```python
from build123d import *

# Parameters (mm, degrees)
BOSS_EXTRUDE1_DEPTH = 6.08
BOSS_EXTRUDE2_DEPTH = 6.09
SKETCH4_W           = 70.899698082
SKETCH4_H           = 9.313865989
CUT_EXTRUDE4_DEPTH  = 13.09
SKETCH5_W           = 29.305939782
SKETCH5_H           = 12.234342693
CUT_EXTRUDE5_DEPTH  = 19.09
SKETCH6_R           = 6
CUT_EXTRUDE6_DEPTH  = 60.839839878
CUT_EXTRUDE7_DEPTH  = 11.09
SKETCH10_W          = 36.097359295
SKETCH10_H          = 22.987225517
CUT_EXTRUDE11_DEPTH = 63.929843377
SKETCH12_W          = 7.8
SKETCH12_H          = 6.08
BOSS_EXTRUDE4_DEPTH = 6
CUT_EXTRUDE12_REACH = 66.913
SKETCH13_W          = 18.746233403
SKETCH13_H          = 9.142839949


with BuildPart() as part:
    # Sketch1 → Boss-Extrude1 (new body)
    with BuildSketch(Plane(origin=(0, 0, 0), x_dir=(1, 0, 0), z_dir=(0, 1, 0))):
        Polygon((-14.914047624, 10.796093069), (-14.914047624, -10.733906931), (57.585952376, -8.821379846), (57.585952376, 8.878620154), align=None)
    extrude(amount=BOSS_EXTRUDE1_DEPTH)

    # Sketch2 → Boss-Extrude2 (add)
    with BuildSketch(Plane(origin=(0, 6.08, 0), x_dir=(1, 0, 0), z_dir=(0, 1, 0))):
        Polygon((-13.064047624, 10.74716445), (-13.064047624, -1.521917904), (57.585952376, 0.341806766), (57.585952376, 8.878620154), align=None)
    extrude(amount=BOSS_EXTRUDE2_DEPTH)

    # Sketch4 → Cut-Extrude4 (cut)
    with BuildSketch(Plane(origin=(0.078934537, 1.089467811, 2.992247256), x_dir=(0.9996522376299903, 0, -0.026370510070028146), z_dir=(0.02478017371916596, 0.34202014332566605, 0.9393658310530242))):
        with Locations((22.35021085, 9.967746424)):
            Rectangle(SKETCH4_W, SKETCH4_H)
    extrude(amount=CUT_EXTRUDE4_DEPTH, mode=Mode.SUBTRACT)

    # Sketch5 → Cut-Extrude5 (cut)
    with BuildSketch(Plane(origin=(52.803749931, 19.218993233, 0), x_dir=(0, 0, -1), z_dir=(0.9396926207859081, 0.34202014332566943, 1.2295842975475839e-15))):
        with Locations((0.411188199, -7.865053205)):
            Rectangle(SKETCH5_W, SKETCH5_H)
    extrude(amount=CUT_EXTRUDE5_DEPTH, mode=Mode.SUBTRACT)

    # Sketch6 → Cut-Extrude6 (cut, through all)
    with BuildSketch(Plane.XZ):
        with Locations((27.215952376, 13.62392238)):
            Circle(SKETCH6_R)
        with Locations((27.215952376, -13.683241685)):
            Circle(SKETCH6_R)
        Polygon((-14.914047624, 10.733906931), (-14.914047624, 8.733906931), (-12.914047624, 10.681147563), align=None)
        Polygon((-14.914047624, -10.796093069), (-12.914047624, -10.743197265), (-14.914047624, -8.796093069), align=None)
        Polygon((55.586647901, 8.874120866), (57.585952376, 8.821379846), (57.585952376, 6.821379846), align=None)
        Polygon((57.585952376, -8.878620154), (57.585952376, -6.878620154), (55.585952376, -8.931515959), align=None)
    extrude(amount=-CUT_EXTRUDE6_DEPTH, mode=Mode.SUBTRACT)

    # Sketch7 → Cut-Extrude7 (cut)
    with BuildSketch(Plane(origin=(0.305261026, 5.260141687, -11.541974951), x_dir=(-0.9997105289622884, 0.009976365195544153, -0.021893615951381312), z_dir=(0.024059473814631405, 0.4145836859950284, -0.9096930850712998))):
        Polygon((-26.921663821, 7.88786599), (-26.921663821, 3.064364781), (-63.575410801, 3.466220434), (-63.575410801, 10.38968732), (-26.921663821, 9.987831666), align=None)
    extrude(amount=CUT_EXTRUDE7_DEPTH, mode=Mode.SUBTRACT)

    # Sketch10 → Cut-Extrude11 (cut, through all)
    with BuildSketch(Plane.ZY.offset(3.214047624)):
        with Locations((0.41938451, 3.731019242)):
            Rectangle(SKETCH10_W, SKETCH10_H)
    extrude(amount=CUT_EXTRUDE11_DEPTH, mode=Mode.SUBTRACT)

    # Sketch12 → Boss-Extrude4 (add)
    with BuildSketch(Plane.ZY.offset(3.214047624)):
        with Locations((-0.030693992, 3.04)):
            Rectangle(SKETCH12_W, SKETCH12_H)
    extrude(amount=BOSS_EXTRUDE4_DEPTH)

    # Sketch13 → Cut-Extrude12 (cut, up to next)
    with BuildSketch(Plane(origin=(-5.91505424, 8.447572923, 0), x_dir=(0, 0, 1), z_dir=(-0.5735764363510444, 0.819152044288993, 0)), mode=Mode.PRIVATE) as cut_extrude12_sk1:
        with Locations((-4.290942315, 4.9788615)):
            Rectangle(SKETCH13_W, SKETCH13_H)
    cut_extrude12_tool1 = extrude(cut_extrude12_sk1.sketch, amount=CUT_EXTRUDE12_REACH, mode=Mode.PRIVATE) & part.part
    add(cut_extrude12_tool1.solids().sort_by_distance((-1.83661, 11.303331, -4.290942))[0], mode=Mode.SUBTRACT)


solid = part.part
```
Model file for the job. Use its own axes, mm. A direction names the side the tool comes from. Coordinates: 2 decimals unless noted, no trailing zeros. Loops run counter-clockwise (first coordinate to the right, second up) from the corner with the lowest first, then second, coordinate; pieces in that order, holes last. Notation, with made-up numbers: (-35.75, 40) - (1.25, 40) arc R26 ccw to (1.25, 57) - close; hole circle Ø5 at (13.25, -7.5). An arc over 180 degrees is marked (long way). Write item = value, one per line. Start each with the question number.
Item 1: Saw through at B-B, the plane y = 5. List the corners of the cut face in (x, z), then the cut area to 3 significant figures.
Item 2: Saw through at A-A, the plane z = -6.25. List the corners of the cut face in (x, y), then the cut area to 3 significant figures.
Item 3: Wall check: probe 1 along Y at (x, z) = (1, 7); probe 2 along X at (y, z) = (3.25, 8.5); probe 3 along Z at (x, y) = (47.5, 3.75). Give the ranges that are in metal, low to high. Write a range as [from, to].
Item 4: 3-axis set-ups, long thin cutter, end or side, ignore diameter. For faces 1 (the face through (-1.888, 11.267, -5.459)), 2 (the face through (-6, 3, 3.869)): which of +Z, -Z, +X, -X, +Y, -Y reach the whole face in a straight line?
Item 5: Pull direction X, two halves, no side cores. Call faces 3 (the face through (-6, 3, -3.931)), 4 (the face through (26.99, 3, 7.63)), 5 (the face through (27.128, 6, -7.684)), 6 (the face through (56.46, 9.17, -4.19)): +X half, -X half, draft (parallel to the pull), parting line (faces both ways), or undercut.
Item 6: Saw through at D-D, the plane z = 0.5. List the corners of the cut face in (x, y).
Item 7: Saw through at C-C, the plane x = -1.5. List the corners of the cut face in (y, z), then the cut area to 3 significant figures.
Item 8: Drop flat-ended pins along their axis: pin 1 Ø1.5 at (x, z) = (35, -6) entering from -Y; pin 2 Ø5 at (x, y) = (28.5, 8) entering from -Z; pin 3 Ø2 at (x, y) = (50, 3.5) entering from -Z; pin 4 Ø4.5 at (x, z) = (22, 3) entering from +Y. Give the stop position or say it passes through.
Answers:
q1.outline = (-9.21, -3.93) - (-3.21, -3.93) - (-3.21, -10.49) - (22.64, -9.8) arc R6 cw to (31.58, -9.57) - (55.59, -8.93) - (57.59, -6.88) - (57.59, 6.82) - (55.59, 8.87) - (31.58, 9.51) arc R6 cw to (22.64, 9.74) - (-3.21, 10.43) - (-3.21, 3.87) - (-9.21, 3.87) - close
q1.area = 1,190 mm2
q2.outline = (-3.21, 0) - (57.59, 0) - (57.59, 6.08) - (55.37, 12.17) - (-0.6, 12.17) - (-3.21, 10.34) - close
q2.area = 731 mm2
q3.probe_1 = [0, 6.08]
q3.probe_2 = [-3.21, 24.09], [30.34, 55.95]
q3.probe_3 = [-9.15, 9.09]
q4.face_1 = +Z, -Z, -X, +Y
q4.face_2 = +Z, -X, +Y, -Y
q5.face_3 = draft
q5.face_4 = undercut
q5.face_5 = undercut
q5.face_6 = +X half
q6.outline = (-9.21, 0) - (57.59, 0) - (57.59, 6.08) - (25.67, 6.08) - (-3.21, 8.17) - (-3.21, 6.08) - (-9.21, 6.08) - close
q7.outline = (0, -10.44) - (11.54, -10.44) - (11.54, -0.77) - (6.08, 1.22) - (6.08, 10.38) - (0, 10.38) - close
q7.area = 185 mm2
q8.pin_1 = 0
q8.pin_2 = -9.03
q8.pin_3 = -9.11
q8.pin_4 = 6.08
